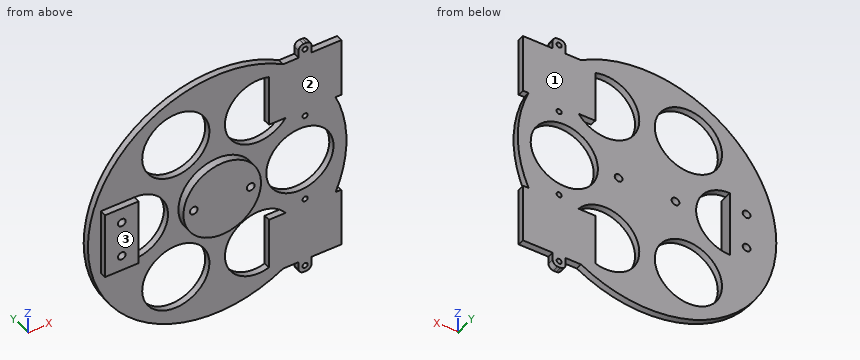
from build123d import *

# Parameters (mm, degrees)
SKETCH_1_R          = 50
EXTRUDE_1_DEPTH     = 2.5
SKETCH_2_R          = 15
EXTRUDE_2_DEPTH     = 3
SKETCH_3_R          = 1.5
CUT_EXTRUDE_1_DEPTH = 71.924255371
SKETCH_5_R          = 13
CUT_EXTRUDE_3_DEPTH = 71.774289117
SKETCH_6_W          = 13
SKETCH_6_H          = 26
EXTRUDE_3_DEPTH     = 2.5
SKETCH_8_R          = 1.5
CUT_EXTRUDE_4_DEPTH = 71.887234394
EXTRUDE_4_DEPTH     = 2.5
SKETCH_11_R         = 1
CUT_EXTRUDE_5_DEPTH = 71.774289117
FILLET_1_R          = 2


with BuildPart() as part:
    # 草图1 → 凸台-拉伸1 (new body)
    with BuildSketch(Plane(origin=(0, 0, 0), x_dir=(1, 0, 0), z_dir=(0, 1, 0))):
        with Locations(Location((0, 0, 0), (0, 0, 270))):
            Circle(SKETCH_1_R)
    extrude(amount=EXTRUDE_1_DEPTH)

    # 草图2 → 凸台-拉伸2 (add)
    with BuildSketch(Plane(origin=(0, 0, 0), x_dir=(-1, 0, 0), z_dir=(0, -1, 0))):
        with Locations(Location((0, 0, 0), (0, 0, 270))):
            Circle(SKETCH_2_R)
    extrude(amount=EXTRUDE_2_DEPTH)

    # 草图3 → 切除-拉伸1 (cut, through all)
    with BuildSketch(Plane(origin=(0, -3, 0), x_dir=(-1, 0, 0), z_dir=(0, -1, 0))):
        with Locations(Location((11, 0, 0), (0, 0, 90))):
            Circle(SKETCH_3_R)
        with Locations(Location((-11, 0, 0), (0, 0, 90))):
            Circle(SKETCH_3_R)
    extrude(amount=-CUT_EXTRUDE_1_DEPTH, mode=Mode.SUBTRACT)

    # 草图5 → 切除-拉伸3 (cut, through all)
    with BuildSketch(Plane(origin=(0, 0, 0), x_dir=(-1, 0, 0), z_dir=(0, -1, 0))):
        with Locations(Location((32, 0, 0), (0, 0, 90))):
            Circle(SKETCH_5_R)
        with Locations(Location((16, -27.712812921, 0), (0, 0, 90))):
            Circle(SKETCH_5_R)
        with Locations(Location((-16, -27.712812921, 0), (0, 0, 90))):
            Circle(SKETCH_5_R)
        with Locations(Location((-32, 0, 0), (0, 0, 90))):
            Circle(SKETCH_5_R)
        with Locations(Location((-16, 27.712812921, 0), (0, 0, 90))):
            Circle(SKETCH_5_R)
        with Locations(Location((16, 27.712812921, 0), (0, 0, 90))):
            Circle(SKETCH_5_R)
    extrude(amount=-CUT_EXTRUDE_3_DEPTH, mode=Mode.SUBTRACT)

    # 草图6 → 凸台-拉伸3 (add, symmetric)
    with BuildSketch(Plane(origin=(0, 0, 0), x_dir=(-1, 0, 0), z_dir=(0, -1, 0))):
        with Locations((38.5, 0)):
            Rectangle(SKETCH_6_W, SKETCH_6_H)
    extrude(amount=EXTRUDE_3_DEPTH, both=True)

    # 草图8 → 切除-拉伸4 (cut, through all)
    with BuildSketch(Plane(origin=(0, -2.5, 0), x_dir=(-1, 0, 0), z_dir=(0, -1, 0))):
        with Locations(Location((38.5, -7, 0), (0, 0, 90))):
            Circle(SKETCH_8_R)
        with Locations(Location((38.5, 7, 0), (0, 0, 90))):
            Circle(SKETCH_8_R)
    extrude(amount=-CUT_EXTRUDE_4_DEPTH, mode=Mode.SUBTRACT)

    # 草图9 → 凸台-拉伸4 (add)
    with BuildSketch(Plane(origin=(0, 0, 0), x_dir=(-1, 0, 0), z_dir=(0, -1, 0))):
        Polygon((-36.5, -43), (-48, -43), (-48, -20), (-20, -20), (-20, -43), (-31.5, -43), (-31.5, -48), (-36.5, -48), align=None)
        Polygon((-31.5, 43), (-31.5, 48), (-36.5, 48), (-36.5, 43), (-48, 43), (-48, 20), (-20, 20), (-20, 43), align=None)
    extrude(amount=-EXTRUDE_4_DEPTH)

    # 草图11 → 切除-拉伸5 (cut, through all)
    with BuildSketch(Plane(origin=(0, 0, 0), x_dir=(-1, 0, 0), z_dir=(0, -1, 0))):
        with Locations(Location((-34, -45.5, 0), (0, 0, 90))):
            Circle(SKETCH_11_R)
        with Locations(Location((-34, -17.5, 0), (0, 0, 90))):
            Circle(SKETCH_11_R)
        with Locations(Location((-34, 17.5, 0), (0, 0, 270))):
            Circle(SKETCH_11_R)
        with Locations(Location((-34, 45.5, 0), (0, 0, 270))):
            Circle(SKETCH_11_R)
    extrude(amount=-CUT_EXTRUDE_5_DEPTH, mode=Mode.SUBTRACT)

    # 圆角1
    fillet_1_edges = [part.edges().sort_by_distance(p)[0] for p in [
        (36.5, 1.25, -48),
        (31.5, 1.25, -48),
        (31.5, 1.25, 48),
        (36.5, 1.25, 48),
    ]]
    fillet(fillet_1_edges, radius=FILLET_1_R)


solid = part.part
The model under review builds one solid part; all positions refer to its coordinate system, in mm. Face numbers are marked on the shaded views. A direction names the side the tool comes from. Round coordinates to 2 decimals unless told otherwise and drop trailing zeros. Loops run counter-clockwise (first coordinate to the right, second up) from the corner with the lowest first, then second, coordinate; pieces in that order, holes last. Notation, with made-up numbers: (-26.75, 6.5) -> (9.25, 6.5) arc R16 ccw to (9.25, 11.5) -> close; hole circle Ø8 at (79.25, -0.5). An arc over 180 degrees is marked (long way). Answer as CSV lines item,"result".
1) Add section C-C on x = -38.5. Write out the cut boundary in (y, z).
Geometry results:
outline,"(-2.5, -13) -> (0, -13) -> (0, -31.9) -> (2.5, -31.9) -> (2.5, -8.5) -> (-2.5, -8.5) -> close; (-2.5, -5.5) -> (2.5, -5.5) -> (2.5, 5.5) -> (-2.5, 5.5) -> close; (-2.5, 8.5) -> (2.5, 8.5) -> (2.5, 31.9) -> (0, 31.9) -> (0, 13) -> (-2.5, 13) -> close"
2) For P1, Ø3, axis at y = 1.5, z = 45, coming from the +X side; P2, Ø0.8, axis at x = 44, y = 1.5, coming from the -Z side; P3, Ø2, axis at x = 24.5, y = 1.5, coming from the +Z side, all flat-tipped, find the tip position at first contact; note any pin that passes through.
Geometry results:
P1,"stops at x = 36.5"
P2,"stops at z = -43"
P3,"stops at z = 44.13"
3) Add section B-B on z = 0. Write out the cut boundary in (x, y), plus the area to 3 significant figures.
Geometry results:
outline,"(-50, 0) -> (-45, 0) -> (-45, -2.5) -> (-32, -2.5) -> (-32, 2.5) -> (-50, 2.5) -> close; (-19, 0) -> (-15, 0) -> (-15, -3) -> (-12.5, -3) -> (-12.5, 2.5) -> (-19, 2.5) -> close; (-9.5, -3) -> (9.5, -3) -> (9.5, 2.5) -> (-9.5, 2.5) -> close; (12.5, -3) -> (15, -3) -> (15, 0) -> (19, 0) -> (19, 2.5) -> (12.5, 2.5) -> close; (45, 0) -> (50, 0) -> (50, 2.5) -> (45, 2.5) -> close"
area,"242 mm²"
4) Add section A-A on y = -1.35. Write out the cut boundary in (x, z).
Geometry results:
outline,"(-45, -13) -> (-32, -13) -> (-32, 13) -> (-45, 13) -> close; circle Ø30 at (0, 0); hole circle Ø3 at (-38.5, -7); hole circle Ø3 at (-38.5, 7); hole circle Ø3 at (-11, 0); hole circle Ø3 at (11, 0)"
5) Tool access review of the marked faces 1, 2 and 3: name each direction out of +Z, -Z, +X, -X, +Y, -Y from which nothing blocks a thin tool from reaching the whole face with its end or side.
Geometry results:
face 1,"+Z, -Z, +X, -X, +Y"
face 2,"-Y"
face 3,"+Z, -Z, -X, -Y"
6) To check wall thickness, follow line 1 along X through (y, z) = (-1, 3); line 2 along X through (y, z) = (1.3, 25); line 3 along Y through (x, z) = (25, -30). State the ranges of each line that lie inside material, in increasing order. Write a range as from..to.
Geometry results:
line 1,"x = -45..-32, -14.7..14.7"
line 2,"x = -43.3..-28.71, -3.29..3.29, 20..48"
line 3,"y = 0..2.5"
7) Add section D-D on x = -24.5. Write out the cut boundary in (y, z), plus the area to 3 significant figures.
Geometry results:
outline,"(0, -43.59) -> (2.5, -43.59) -> (2.5, -37.55) -> (0, -37.55) -> close; (0, -17.88) -> (2.5, -17.88) -> (2.5, -10.62) -> (0, -10.62) -> close; (0, 10.62) -> (2.5, 10.62) -> (2.5, 17.88) -> (0, 17.88) -> close; (0, 37.55) -> (2.5, 37.55) -> (2.5, 43.59) -> (0, 43.59) -> close"
area,"66.5 mm²"
